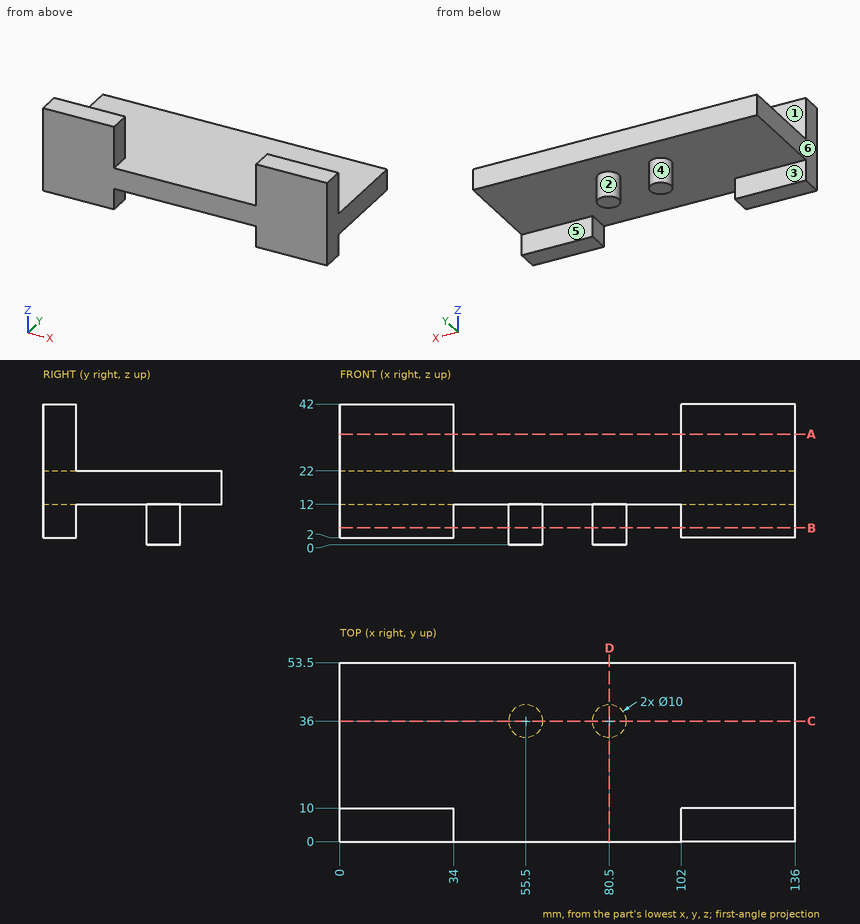
Input: dimensioned drawing with shaded views. Units: mm. Origin: part minimum x, y, z. A direction names the side the tool comes from. Give positions to 0.01 mm unless a question says otherwise; leave off trailing zeros. Write each loop counter-clockwise with the first axis right and the second up, starting at its lowest first coordinate (ties: lowest second). Pieces come first, ordered by that corner, then holes.
1. Access query for the marked faces 1, 2 and 3. Directions: +Z, -Z, +X, -X, +Y, -Y. A direction counts if a zero-diameter tool reaches every point of the face in a straight line with its end or side. Return the directions, or none.
2. Section query C-C (y = 36). Return the cut outline in (x, z).
3. Pull-direction query (X, two-part tool) for the marked faces 4, 5 and 6; classes: +X half, -X half, draft (parallel to the pull), parting line (faces both ways), or undercut.
4. Section query B-B (z = 5). Return the cut outline in (x, y).
5. Section query A-A (z = 33). Return the cut outline in (x, y), then the cut area to 3 significant figures.
6. Section query D-D (x = 80.5). Return the cut outline in (y, z).
7. Material intervals for line 1 along Y through (x, z) = (20.5, 6); line 2 along Z through (x, y) = (8.5, 33); line 3 along Z through (x, y) = (25.5, 8), sorted ascending.
8. First-contact query: pin 1 (5 mm diameter, centred on x = 121.5, z = 8.5, fed in from +Y); pin 2 (4 mm diameter, centred on x = 22, y = 13.5, fed in from +Z); pin 3 (11 mm diameter, centred on x = 24.5, y = 6.5, fed in from -Z). Flat tips, straight axial feed; report the tip coordinate or a pass-through.
Output values:
1. face 1: +Z, +X, -X, +Y
1. face 2: -Z
1. face 3: -Z, +X, -X, +Y
2. outline: (0, 12) - (50.5, 12) - (50.5, 0) - (60.5, 0) - (60.5, 12) - (75.5, 12) - (75.5, 0) - (85.5, 0) - (85.5, 12) - (136, 12) - (136, 22) - (0, 22) - close
3. face 4: undercut
3. face 5: draft
3. face 6: -X half
4. outline: (0, 0) - (34, 0) - (34, 10) - (0, 10) - close; circle Ø10 at (55.5, 36); circle Ø10 at (80.5, 36); (102, 0) - (136, 0) - (136, 10) - (102, 10) - close
5. outline: (0, 0) - (34, 0) - (34, 10) - (0, 10) - close; (102, 0) - (136, 0) - (136, 10) - (102, 10) - close
5. area: 680 mm2
6. outline: (0, 12) - (31, 12) - (31, 0) - (41, 0) - (41, 12) - (53.5, 12) - (53.5, 22) - (0, 22) - close
7. line 1: y = 0 to 10
7. line 2: z = 12 to 22
7. line 3: z = 2 to 42
8. pin 1: stops at y = 10
8. pin 2: stops at z = 22
8. pin 3: stops at z = 2
